Answer from the drawing. Dimensions are ordinates in mm from the lowest x, y and z of the part. Coordinates: 2 decimals unless noted, no trailing zeros. Order: outer loops, then holes, each group sorted by start corner. A loop starts at its lowest first (then second) coordinate and runs counter-clockwise, first axis right, second up. Notation, with made-up numbers: (31.25, 2) -> (67.25, 2) arc R18 cw to (67.25, 20) -> close; hole circle Ø8 at (53, 16). An arc over 180 degrees is marked (long way). Answer as a JSON object with one key per item and string values. Group by question number.
1) Consider L1, parallel to X at y = 60.5, z = 1.3; L2, parallel to X at y = 119, z = 1.2 (1 decimal); L3, parallel to Y at x = 155, z = 0.85. Determine where each line is inside the solid, lowest interval first.
2) Section C-C on y = 144 is taken. Determine the outline of the cut face in (x, z).
3) Section B-B on x = 25 is taken. Determine the outline of the cut face in (y, z).
4) Section A-A on z = 0.35 is taken. Determine the outline of the cut face in (x, y).
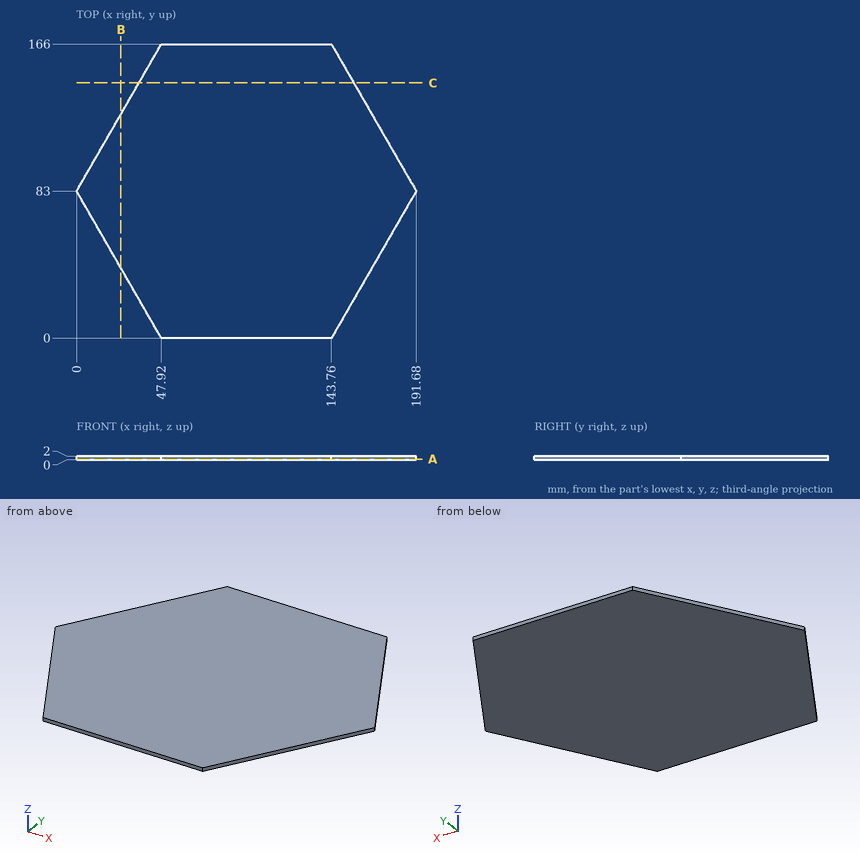
Worked answers:
{
 "1": {"L1": "x = 12.99 to 178.69", "L2": "x = 20.8 to 170.9", "L3": "y = 19.47 to 146.53"},
 "2": {"outline": "(35.22, 0) -> (156.46, 0) -> (156.46, 2) -> (35.22, 2) -> close"},
 "3": {"outline": "(39.7, 0) -> (126.3, 0) -> (126.3, 2) -> (39.7, 2) -> close"},
 "4": {"outline": "(0, 83) -> (47.92, 0) -> (143.76, 0) -> (191.68, 83) -> (143.76, 166) -> (47.92, 166) -> close"}
}
